Could you check a few things on this model? Use its own coordinates, in mm. Face numbers are marked on the shaded views. A direction names the side the tool comes from. Coordinates: 2 decimals unless noted, no trailing zeros. Write each loop counter-clockwise with the first axis right and the second up, starting at its lowest first coordinate (ties: lowest second). Pieces come first, ordered by that corner, then holes. Notation, with made-up numbers: (8.25, -35.5) - (61.25, -35.5) arc R18 ccw to (61.25, -18.5) - close; hole circle Ø2 at (20, 15). An arc over 180 degrees is marked (long way). Answer as a JSON object with one key per item and string values. Group by question number.
1) If we section it at D-D (x = -13.5): Write out the boundary of the cut face in (y, z), plus the area to 3 significant figures.
2) If we section it at A-A (x = 2.5): Write out the boundary of the cut face in (y, z), plus the area to 3 significant figures.
3) If we section it at B-B (z = 13.75): Write out the boundary of the cut face in (x, y).
4) If we section it at C-C (y = 1): Write out the boundary of the cut face in (x, z).
5) On a 3-axis mill with a long thin cutter (end or side, diameter ignored), from which of +Z, -Z, +X, -X, +Y, -Y can I reach the whole of each face in a straight line? I mean the marked faces 1 and 2. Say none if no direction works.
6) Will these pins go through, and if not, where does the flat tip stop? pin 1 Ø0.7 at (x, y) = (-16.5, -30) entering from +Z; pin 2 Ø0.6 at (y, z) = (34, 16) entering from +X.
7) Please list where these lines run through material, in increasing order: line 1 along X through (y, z) = (4, 2.75); line 2 along Y through (x, z) = (12, 4.5); line 3 along X through (y, z) = (31.5, 4).
8) We'd pull the mould along X, two halves only. Please class the marked faces 3, 4 and 5: released by +X, released by -X, zero draft, split by the parting line, or undercut.
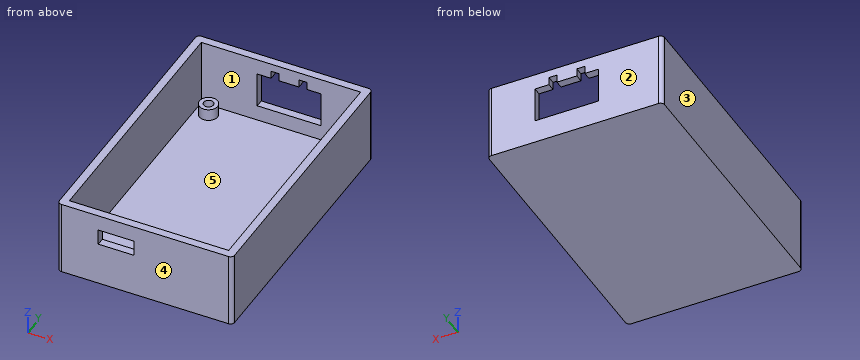
```python
from build123d import *

# Parameters (mm, degrees)
F0_W     = 40
F0_H     = 65
F0_R     = 2.2837988166
F0_R_2   = 1.2192556023
F1_DEPTH = 2
F2_DEPTH = 19
F3_DEPTH = 5
F5_DEPTH = 5
F6_W     = 9
F6_H     = 4
F7_DEPTH = 5


with BuildPart() as f1:
    # F0 (on Top) → F1 (new body)
    with BuildSketch(Plane.XY):
        with BuildLine():
            ThreePointArc((22, 33.5), (21.7071067812, 34.2071067812), (21, 34.5))
            Line((21, 34.5), (-21, 34.5))
            ThreePointArc((-21, 34.5), (-21.7071067812, 34.2071067812), (-22, 33.5))
            Line((-22, 33.5), (-22, -33.5))
            ThreePointArc((-22, -33.5), (-21.7071067812, -34.2071067812), (-21, -34.5))
            Line((-21, -34.5), (21, -34.5))
            ThreePointArc((21, -34.5), (21.7071067812, -34.2071067812), (22, -33.5))
            Line((22, -33.5), (22, 33.5))
        make_face()
        Rectangle(F0_W, F0_H, mode=Mode.SUBTRACT)
        Rectangle(F0_W, F0_H)
        with Locations((-16.6275631636, -29.5829899758)):
            Circle(F0_R, mode=Mode.SUBTRACT)
        with Locations((17.0274368364, -29.5829899758)):
            Circle(F0_R, mode=Mode.SUBTRACT)
        with Locations((-16.6275631636, 29.4170100242)):
            Circle(F0_R, mode=Mode.SUBTRACT)
        with Locations((17.0274368364, 29.4170100242)):
            Circle(F0_R, mode=Mode.SUBTRACT)
        with Locations((17.0274368364, -29.5829899758)):
            Circle(F0_R)
        with Locations((17.0274368364, -29.5829899758)):
            Circle(F0_R_2, mode=Mode.SUBTRACT)
        with Locations((-16.6275631636, -29.5829899758)):
            Circle(F0_R)
        with Locations((-16.6275631636, -29.5829899758)):
            Circle(F0_R_2, mode=Mode.SUBTRACT)
        with Locations((17.0274368364, 29.4170100242)):
            Circle(F0_R)
        with Locations((17.0274368364, 29.4170100242)):
            Circle(F0_R_2, mode=Mode.SUBTRACT)
        with Locations((-16.6275631636, 29.4170100242)):
            Circle(F0_R)
        with Locations((-16.6275631636, 29.4170100242)):
            Circle(F0_R_2, mode=Mode.SUBTRACT)
        with Locations((-16.6275631636, -29.5829899758)):
            Circle(F0_R_2)
        with Locations((17.0274368364, -29.5829899758)):
            Circle(F0_R_2)
        with Locations((17.0274368364, 29.4170100242)):
            Circle(F0_R_2)
        with Locations((-16.6275631636, 29.4170100242)):
            Circle(F0_R_2)
    extrude(amount=F1_DEPTH)

    # F0 (on Top) → F2 (join)
    with BuildSketch(Plane.XY):
        with BuildLine():
            ThreePointArc((22, 33.5), (21.7071067812, 34.2071067812), (21, 34.5))
            Line((21, 34.5), (-21, 34.5))
            ThreePointArc((-21, 34.5), (-21.7071067812, 34.2071067812), (-22, 33.5))
            Line((-22, 33.5), (-22, -33.5))
            ThreePointArc((-22, -33.5), (-21.7071067812, -34.2071067812), (-21, -34.5))
            Line((-21, -34.5), (21, -34.5))
            ThreePointArc((21, -34.5), (21.7071067812, -34.2071067812), (22, -33.5))
            Line((22, -33.5), (22, 33.5))
        make_face()
        Rectangle(F0_W, F0_H, mode=Mode.SUBTRACT)
    extrude(amount=F2_DEPTH)

    # F0 (on Top) → F3 (join)
    with BuildSketch(Plane.XY):
        with Locations((-16.6275631636, 29.4170100242)):
            Circle(F0_R)
        with Locations((-16.6275631636, 29.4170100242)):
            Circle(F0_R_2, mode=Mode.SUBTRACT)
        with Locations((17.0274368364, 29.4170100242)):
            Circle(F0_R)
        with Locations((17.0274368364, 29.4170100242)):
            Circle(F0_R_2, mode=Mode.SUBTRACT)
        with Locations((-16.6275631636, -29.5829899758)):
            Circle(F0_R)
        with Locations((-16.6275631636, -29.5829899758)):
            Circle(F0_R_2, mode=Mode.SUBTRACT)
        with Locations((17.0274368364, -29.5829899758)):
            Circle(F0_R)
        with Locations((17.0274368364, -29.5829899758)):
            Circle(F0_R_2, mode=Mode.SUBTRACT)
    extrude(amount=F3_DEPTH)

    # F4 (on face) → F5 (cut)
    with BuildSketch(Plane(origin=(0, 34.5, 0), x_dir=(-1, 0, 0), z_dir=(0, 1, 0))):
        Polygon((-10.027, 6), (5.973, 6), (5.973, 15), (2.473, 15), (2.473, 17), (0.473, 17), (0.473, 15), (-4.527, 15), (-4.527, 17), (-6.527, 17), (-6.527, 15), (-10.027, 15), align=None)
    extrude(amount=-F5_DEPTH, mode=Mode.SUBTRACT)

    # F6 (on face) → F7 (cut)
    with BuildSketch(Plane.XZ.offset(34.5)):
        with Locations((-7.2275631636, 13)):
            Rectangle(F6_W, F6_H)
    extrude(amount=-F7_DEPTH, mode=Mode.SUBTRACT)


solid = f1.part
```
Here are the results:
{
 "1": {"outline": "(-34.5, 0) - (34.5, 0) - (34.5, 19) - (32.5, 19) - (32.5, 2) - (-32.5, 2) - (-32.5, 19) - (-34.5, 19) - close", "area": "206 mm²"},
 "2": {"outline": "(-34.5, 0) - (34.5, 0) - (34.5, 6) - (32.5, 6) - (32.5, 2) - (-32.5, 2) - (-32.5, 19) - (-34.5, 19) - close; (32.5, 15) - (34.5, 15) - (34.5, 19) - (32.5, 19) - close", "area": "188 mm²"},
 "3": {"outline": "(-22, -33.5) arc R1 ccw to (-21, -34.5) - (-11.73, -34.5) - (-11.73, -32.5) - (-20, -32.5) - (-20, 32.5) - (-5.97, 32.5) - (-5.97, 34.5) - (-21, 34.5) arc R1 ccw to (-22, 33.5) - close; (-2.73, -34.5) - (21, -34.5) arc R1 ccw to (22, -33.5) - (22, 33.5) arc R1 ccw to (21, 34.5) - (10.03, 34.5) - (10.03, 32.5) - (20, 32.5) - (20, -32.5) - (-2.73, -32.5) - close"},
 "4": {"outline": "(-22, 0) - (22, 0) - (22, 19) - (20, 19) - (20, 2) - (-20, 2) - (-20, 19) - (-22, 19) - close"},
 "5": {"face 1": "+Z", "face 2": "+Z, -Z, +X, -X, +Y"},
 "6": {"pin 1": "stops at z = 2", "pin 2": "stops at x = 21.98"},
 "7": {"line 1": "x = -22 to -20, 20 to 22", "line 2": "y = -34.5 to -32.5, 32.5 to 34.5", "line 3": "x = -22 to -20, -17.56 to -15.69, 16.09 to 17.96, 20 to 22"},
 "8": {"face 3": "released by -X", "face 4": "zero draft", "face 5": "undercut"}
}
